The model under review builds one solid part; all positions refer to its coordinate system, in mm. Face numbers are marked on the shaded views. A direction names the side the tool comes from. Give positions to 0.01 mm unless a question says otherwise; leave off trailing zeros. Order: outer loops, then holes, each group sorted by start corner. A loop starts at its lowest first (then second) coordinate and runs counter-clockwise, first axis right, second up.
```python
from build123d import *

# Parameters (mm, degrees)
F0_W     = 39.6875
F0_H     = 25.4
F1_DEPTH = 6.35
F2_W     = 12.7
F2_H     = 6.35
F3_DEPTH = 2
F4_R     = 1.5875
F5_DEPTH = 25.4


with BuildPart() as f1:
    # F0 (on Top) → F1 (new body)
    with BuildSketch(Plane.XY):
        with Locations((19.84375, 12.7)):
            Rectangle(F0_W, F0_H)
    extrude(amount=F1_DEPTH)

    # F2 (on face) → F3 (cut)
    with BuildSketch(Plane(origin=(0, 0, 0), x_dir=(0, -1, 0), z_dir=(-1, 0, 0))):
        with Locations((-6.35, 3.175)):
            Rectangle(F2_W, F2_H)
    extrude(amount=-F3_DEPTH, mode=Mode.SUBTRACT)

    # F4 (on face) → F5 (cut)
    with BuildSketch(Plane.XY.offset(6.35)):
        with Locations((33.3375, 12.7)):
            Circle(F4_R)
    extrude(amount=-F5_DEPTH, mode=Mode.SUBTRACT)


solid = f1.part
```
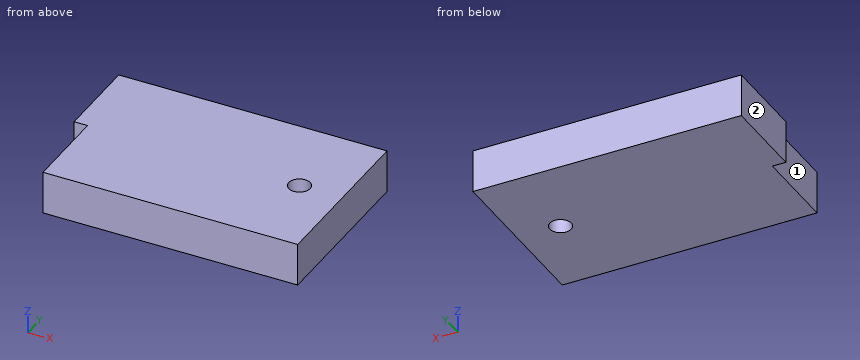
Item 1: Clearance check with flat-ended pins moving along their axes: pin 1 Ø1 at (x, z) = (30.5, 2.5) entering from -Y; pin 2 Ø1 at (x, z) = (0.5, 2.5) entering from -Y. State where each tip first meets the part, or that it passes through.
Values found:
pin 1: stops at y = 0
pin 2: stops at y = 12.7
Item 2: Take a section at A-A (z = 1.5). Give the boundary of the cut face in (x, y) (1 decimal).
Values found:
outline: (0, 12.7) - (2, 12.7) - (2, 0) - (39.7, 0) - (39.7, 25.4) - (0, 25.4) - close; hole circle Ø3.2 at (33.3, 12.7)
Item 3: For the marked faces 1 and 2, list the 3-axis set-ups (+Z, -Z, +X, -X, +Y, -Y) from which the entire face can be reached by the end or side of a thin tool; tool diameter is ignored.
Values found:
face 1: +Z, -Z, -X, -Y
face 2: +Z, -Z, -X, +Y, -Y
Item 4: For line 1 (X direction, y = 8.25, z = 5.5), list the stretches that pass through material, from the lowest coordinate up.
Values found:
line 1: x = 2 to 39.69
Item 5: Take a section at B-B (y = 13.25). Give the boundary of the cut face in (x, z).
Values found:
outline: (0, 0) - (31.85, 0) - (31.85, 6.35) - (0, 6.35) - close; (34.83, 0) - (39.69, 0) - (39.69, 6.35) - (34.83, 6.35) - close
Item 6: Take a section at C-C (y = 2.75). Give the boundary of the cut face in (x, z), and give its area (3 significant figures).
Values found:
outline: (2, 0) - (39.69, 0) - (39.69, 6.35) - (2, 6.35) - close
area: 239 mm2
